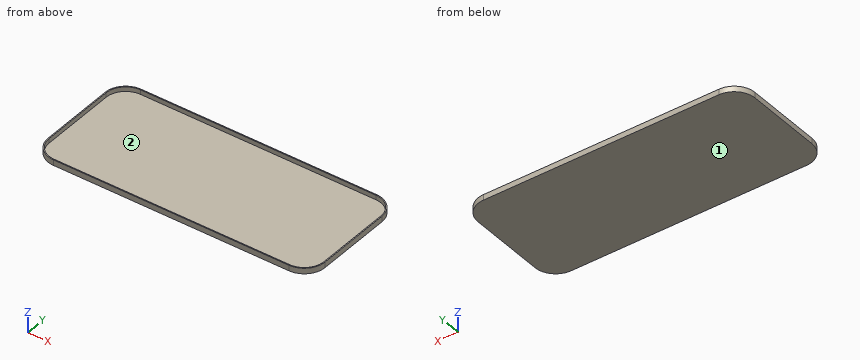
from build123d import *

# Parameters (mm, degrees)
F0_W     = 200
F0_H     = 85
F1_DEPTH = 4
F2_R     = 15
F3_T     = -0.75


with BuildPart() as f1:
    # F0 (on Top) → F1 (new body)
    with BuildSketch(Plane.XY):
        with Locations((100, 42.5)):
            Rectangle(F0_W, F0_H)
    extrude(amount=-F1_DEPTH)

    # F2
    f2_edges = [f1.edges().sort_by_distance(p)[0] for p in [
        (0, 0, -2),
        (200, 0, -2),
        (200, 85, -2),
        (0, 85, -2),
    ]]
    fillet(f2_edges, radius=F2_R)

    # F3
    f3_openings = [f1.faces().sort_by_distance(p)[0] for p in [
        (100, 42.5, 0),
    ]]
    offset(amount=F3_T, openings=f3_openings)


solid = f1.part
Model file for the job. Use its own axes, mm. Face numbers are marked on the shaded views. Give positions to 0.01 mm unless a question says otherwise; leave off trailing zeros. Order: outer loops, then holes, each group sorted by start corner. A loop starts at its lowest first (then second) coordinate and runs counter-clockwise, first axis right, second up. Notation, with made-up numbers: (87.25, 85.5) - (115.25, 85.5) arc R27 cw to (115.25, 107.5) - close; hole circle Ø10 at (9, 56.5). An arc over 180 degrees is marked (long way). Return JSON: item names as keys, results as strings.
1) Pull direction Y, two halves, no side cores. Call the marked faces 1 and 2: pulls with the +Y half, pulls with the -Y half, needs draft (parallel to the pull), parting line crosses it, or undercut.
Geometry says:
{"face 1": "needs draft", "face 2": "undercut"}
2) Flat gauge pin, fed straight in: P1, Ø3, axis at x = 39.5, y = 70.5, coming from the +Z side. Where does the tip first touch, or does it go through?
Geometry says:
{"P1": "z = -3.25"}
3) Probe line 1 (Y direction, x = 156, z = -0.15); line 2 (X direction, y = 38.5, z = -1.6); line 3 (Z direction, x = 108, y = 79). List the from-to ranges inside material, lowest first. Write a range as from..to.
Geometry says:
{"line 1": "0..0.75, 84.25..85", "line 2": "0..0.75, 199.25..200", "line 3": "-4..-3.25"}
4) Cut at B-B, the plane y = 39. Give the cut face in (x, z), plus the area to 3 significant figures.
Geometry says:
{"outline": "(0, -4) - (200, -4) - (200, 0) - (199.25, 0) - (199.25, -3.25) - (0.75, -3.25) - (0.75, 0) - (0, 0) - close", "area": "155 mm²"}
5) Cut at C-C, the plane x = 40. Give the cut face in (y, z).
Geometry says:
{"outline": "(0, -4) - (85, -4) - (85, 0) - (84.25, 0) - (84.25, -3.25) - (0.75, -3.25) - (0.75, 0) - (0, 0) - close"}
6) Cut at A-A, the plane z = -2.15. Give the cut face in (x, y), plus the area to 3 significant figures.
Geometry says:
{"outline": "(0, 15) arc R15 ccw to (15, 0) - (185, 0) arc R15 ccw to (200, 15) - (200, 70) arc R15 ccw to (185, 85) - (15, 85) arc R15 ccw to (0, 70) - close; hole (0.75, 15) arc R14.25 ccw to (15, 0.75) - (185, 0.75) arc R14.25 ccw to (199.25, 15) - (199.25, 70) arc R14.25 ccw to (185, 84.25) - (15, 84.25) arc R14.25 ccw to (0.75, 70) - close", "area": "406 mm²"}
